from build123d import *

# Parameters (mm, degrees)
F0_W     = 42
F0_H     = 42
F1_DEPTH = 887
F2_W     = 21
F2_H     = 41.604375
F3_DEPTH = 42
F4_W     = 18
F4_H     = 17
F5_DEPTH = 42


with BuildPart() as f1:
    # F0 (on Top) → F1 (new body)
    with BuildSketch(Plane.XY):
        with Locations((-34.786186, 16.720576)):
            Rectangle(F0_W, F0_H)
    extrude(amount=F1_DEPTH)

    # F2 (on face) → F3 (cut)
    with BuildSketch(Plane.YZ.offset(-13.786186)):
        with Locations((6.220576, 866.197813)):
            Rectangle(F2_W, F2_H)
    extrude(amount=-F3_DEPTH, mode=Mode.SUBTRACT)

    # F4 (on face) → F5 (cut)
    with BuildSketch(Plane.YZ.offset(-13.786186)):
        with Locations((4.720576, 594.488045)):
            Rectangle(F4_W, F4_H)
    extrude(amount=-F5_DEPTH, mode=Mode.SUBTRACT)


solid = f1.part
Check sheet for the modelled part. Datum: model origin and axes. Units: mm. A direction names the side the tool comes from. Coordinates: 2 decimals unless noted, no trailing zeros. Write each loop counter-clockwise with the first axis right and the second up, starting at its lowest first coordinate (ties: lowest second). Pieces come first, ordered by that corner, then holes.
Item 1: Mould release check, pull along Z, two halves, no side actions. Record for faces 1 (the face through (-34, 16.721, 866)), 2 (the face through (-34, 6, 845.396)), 3 (the face through (-34, 5, 585.988)), 4 (the face through (-35, 17, 0)): released by +Z, released by -Z, zero draft, split by the parting line, or undercut.
Numbers:
face 1: zero draft
face 2: released by +Z
face 3: undercut
face 4: released by -Z
Item 2: Access from +Z, -Z, +X, -X, +Y, -Y to the whole of each face (thin tool, end or side, straight path). Record for faces 5 (the face through (-13.786, 16, 437)), 6 (the face through (-34, 13.721, 594)).
Numbers:
face 5: +Z, -Z, +X, +Y, -Y
face 6: +X, -X, -Y
Item 3: Cross-section at A-A on x = -28.5. Record the boundary of the cut face in (y, z).
Numbers:
outline: (-4.28, 0) - (37.72, 0) - (37.72, 887) - (16.72, 887) - (16.72, 845.4) - (-4.28, 845.4) - (-4.28, 602.99) - (13.72, 602.99) - (13.72, 585.99) - (-4.28, 585.99) - close
Item 4: Depth check by flat-ended pin: pin 1 Ø21 at (x, z) = (-30, 856.5) entering from -Y; pin 2 Ø10.5 at (x, y) = (-37.5, 3.5) entering from +Z; pin 3 Ø5 at (x, z) = (-43.5, 592) entering from -Y. Enter the tip coordinate at first touch or a pass-through.
Numbers:
pin 1: stops at y = 16.72
pin 2: stops at z = 845.4
pin 3: stops at y = 13.72
Item 5: Scan lines: probe 1 along Z at (x, y) = (-20.5, 9); probe 2 along Y at (x, z) = (-45.5, 601.5); probe 3 along Z at (x, y) = (-37.5, 16.5). Record each from-to range of solid material in increasing order.
Numbers:
probe 1: z = 0 to 585.99, 602.99 to 845.4
probe 2: y = 13.72 to 37.72
probe 3: z = 0 to 845.4
